```python
from build123d import *

# Parameters (mm, degrees)
SKETCH1_W                  = 91
SKETCH1_H                  = 62
BOSS_EXTRUDE1_DEPTH        = 6
SKETCH2_W                  = 85.4
SKETCH2_H                  = 56.4
CUT_EXTRUDE1_DEPTH         = 4
SKETCH3_R                  = 3
SKETCH3_R_2                = 1.4
BOSS_EXTRUDE2_DEPTH        = 2
CHAMFER1_SIZE              = 1
CHAMFER2_SIZE              = 0.4
LPATTERN1_COUNT            = 2
LPATTERN1_PITCH            = 58
LPATTERN1_COUNT_DIR2       = 2
LPATTERN1_PITCH_DIR2       = 49
CHAMFER1_OF_LPATTERN1_SIZE = 1


with BuildPart() as part:
    # Sketch1 → Boss-Extrude1 (new body)
    with BuildSketch(Plane.XY):
        Rectangle(SKETCH1_W, SKETCH1_H)
    extrude(amount=BOSS_EXTRUDE1_DEPTH)

    # Sketch2 → Cut-Extrude1 (cut)
    with BuildSketch(Plane.XY.offset(6)):
        Rectangle(SKETCH2_W, SKETCH2_H)
    extrude(amount=-CUT_EXTRUDE1_DEPTH, mode=Mode.SUBTRACT)

    # Sketch3 → Boss-Extrude2 (add)
    with BuildSketch(Plane.XY.offset(2)):
        with Locations(Location((-39, 24.5, 0), (0, 0, 180))):
            Circle(SKETCH3_R)
        with Locations((-39, 24.5)):
            Circle(SKETCH3_R_2, mode=Mode.SUBTRACT)
    boss_extrude2 = extrude(amount=BOSS_EXTRUDE2_DEPTH)

    # Chamfer1
    # the kernel refuses this chamfer: 1 mm, written as the material it adds along each edge
    with BuildSketch(Plane(origin=(-39, 24.5, 2), x_dir=(-1, 0, 0), z_dir=(0, 1, 0))) as chamfer1_piece_1:
        Polygon((3 + CHAMFER1_SIZE, 0), (3, CHAMFER1_SIZE), (3, 0), align=None)
    revolve(axis=Axis((-39, 24.5, 2), (0, 0, 1)))

    # Chamfer2
    chamfer2_edges = [part.edges().sort_by_distance(p)[0] for p in [
        (42.7, 0, 6),
        (0, 28.2, 6),
        (-42.7, 0, 6),
        (0, -28.2, 6),
    ]]
    chamfer(chamfer2_edges, length=CHAMFER2_SIZE)

    # LPattern1: Boss-Extrude2 2 × 2
    with Locations(*[(i * LPATTERN1_PITCH, -j * LPATTERN1_PITCH_DIR2, 0) for i in range(LPATTERN1_COUNT) for j in range(LPATTERN1_COUNT_DIR2) if (i, j) != (0, 0)]):
        add(boss_extrude2)

    # Chamfer1 of LPattern1
    # the kernel refuses this chamfer: 1 mm, written as the material it adds along each edge
    with BuildSketch(Plane(origin=(-39, -24.5, 2), x_dir=(-1, 0, 0), z_dir=(0, 1, 0))) as chamfer1_of_lpattern1_piece_1:
        Polygon((3 + CHAMFER1_OF_LPATTERN1_SIZE, 0), (3, CHAMFER1_OF_LPATTERN1_SIZE), (3, 0), align=None)
    revolve(axis=Axis((-39, -24.5, 2), (0, 0, 1)))
    with BuildSketch(Plane(origin=(19, 24.5, 2), x_dir=(-1, 0, 0), z_dir=(0, 1, 0))) as chamfer1_of_lpattern1_piece_2:
        Polygon((3 + CHAMFER1_OF_LPATTERN1_SIZE, 0), (3, CHAMFER1_OF_LPATTERN1_SIZE), (3, 0), align=None)
    revolve(axis=Axis((19, 24.5, 2), (0, 0, 1)))
    with BuildSketch(Plane(origin=(19, -24.5, 2), x_dir=(-1, 0, 0), z_dir=(0, 1, 0))) as chamfer1_of_lpattern1_piece_3:
        Polygon((3 + CHAMFER1_OF_LPATTERN1_SIZE, 0), (3, CHAMFER1_OF_LPATTERN1_SIZE), (3, 0), align=None)
    revolve(axis=Axis((19, -24.5, 2), (0, 0, 1)))


solid = part.part
```
CAD build for the part. Positions are in the model's coordinates, mm. A direction names the side the tool comes from. Coordinates: 2 decimals unless noted, no trailing zeros. Loops run counter-clockwise (first coordinate to the right, second up) from the corner with the lowest first, then second, coordinate; pieces in that order, holes last. Notation, with made-up numbers: (56, 76) - (63, 76) arc R31 ccw to (63, 104) - close; hole circle Ø10 at (67.5, 83.5). An arc over 180 degrees is marked (long way). Use CSV: the item, a comma, the result in double quotes. Start each with the question number.
Q1. Drop flat-ended pins along their axis: P1, Ø0.8, axis at x = 19, y = -24, coming from the +Z side; P2, Ø0.7, axis at x = -41.5, y = -27, coming from the +Z side; P3, Ø3, axis at x = 20, y = -25, coming from the +Z side. Give the stop position or say it passes through.
Q2. 3-axis set-ups, long thin cutter, end or side, ignore diameter. For faces 1 (the flat face through (-42, 28, 2)), 2 (the flat face through (45.5, 0, 3)): which of +Z, -Z, +X, -X, +Y, -Y reach the whole face in a straight line?
Q3. Cut at C-C, the plane x = 19. List the corners of the cut face in (y, z).
Q4. Probe probe 1 along Y at (x, z) = (19, 3.15); probe 2 along X at (y, z) = (8, 4.25); probe 3 along X at (y, z) = (-27, 2.75). List the from-to ranges inside material, lowest first. Write a range as from..to.
Q5. Two-plate mould, pull along Y, no slides. Class faces 3 (the flat face through (-1, 28.2, 4)), 4 (the flat face through (-1, -31, 3)), 5 (the flat face through (-1, 0, 0)), 6 (the flat face through (-40, 26, 4)): +Y half, -Y half, draft (parallel to the pull), parting line (faces both ways), or undercut.
Q6. Cut at A-A, the plane x = 9. List the corners of the cut face in (y, z).
Q7. Cut at B-B, the plane y = 17. List the corners of the cut face in (x, z).
Here are the results:
1,P1,"z = 2"
1,P2,"z = 2.81"
1,P3,"z = 4"
2,face 1,"+Z"
2,face 2,"+Z, -Z, +X, +Y, -Y"
3,outline,"(-31, 0) - (31, 0) - (31, 6) - (28.6, 6) - (28.2, 5.6) - (28.2, 2.3) - (27.5, 3) - (27.5, 4) - (25.9, 4) - (25.9, 2) - (23.1, 2) - (23.1, 4) - (21.5, 4) - (21.5, 3) - (20.5, 2) - (-20.5, 2) - (-21.5, 3) - (-21.5, 4) - (-23.1, 4) - (-23.1, 2) - (-25.9, 2) - (-25.9, 4) - (-27.5, 4) - (-27.5, 3) - (-28.2, 2.3) - (-28.2, 5.6) - (-28.6, 6) - (-31, 6) - close"
4,probe 1,"-31..-28.2, -27.5..-25.9, -23.1..-21.5, 21.5..23.1, 25.9..27.5, 28.2..31"
4,probe 2,"-45.5..-42.7, 42.7..45.5"
4,probe 3,"-45.5..-42.7, -41.08..-36.92, 16.92..21.08, 42.7..45.5"
5,face 3,"undercut"
5,face 4,"-Y half"
5,face 5,"draft"
5,face 6,"undercut"
6,outline,"(-31, 0) - (31, 0) - (31, 6) - (28.6, 6) - (28.2, 5.6) - (28.2, 2) - (-28.2, 2) - (-28.2, 5.6) - (-28.6, 6) - (-31, 6) - close"
7,outline,"(-45.5, 0) - (45.5, 0) - (45.5, 6) - (43.1, 6) - (42.7, 5.6) - (42.7, 2) - (-42.7, 2) - (-42.7, 5.6) - (-43.1, 6) - (-45.5, 6) - close"
